from build123d import *

# Parameters (mm, degrees)
SKETCH3_R = 0.5


with BuildPart() as part:
    # Sweep2: sweep along a path in Sketch1
    with BuildLine(Plane(origin=(0, 0, 0), x_dir=(0, 0, -1), z_dir=(1, 0, 0))) as sweep2_path:
        Line((16, 4), (14, 4))
        ThreePointArc((14, 4), (13.292893219, 3.707106781), (13, 3))
        Line((13, 3), (13, 1))
        ThreePointArc((13, 1), (12.707106781, 0.292893219), (12, 0))
        Line((12, 0), (-12, 0))
        ThreePointArc((-12, 0), (-12.707106781, 0.292893219), (-13, 1))
        Line((-13, 1), (-13, 7))
        ThreePointArc((-13, 7), (-12.707106781, 7.707106781), (-12, 8))
        Line((-12, 8), (-6, 8))
    # Sketch3 → Sweep2 (sweep)
    with BuildSketch(Plane.XY):
        Circle(SKETCH3_R)
    sweep(path=sweep2_path.line)


solid = part.part
Work out the finished part from the listing and answer in its coordinate system (mm). A direction names the side the tool comes from. Give positions to 0.01 mm unless a question says otherwise; leave off trailing zeros. Order: outer loops, then holes, each group sorted by start corner. A loop starts at its lowest first (then second) coordinate and runs counter-clockwise, first axis right, second up. Notation, with made-up numbers: (68, -21) -> (95, -21) arc R26 ccw to (95, 6) -> close; hole circle Ø4 at (0, 46). An arc over 180 degrees is marked (long way). Answer as a JSON object with one key per item and string values. Group by question number.
1. Section B-B on y = 1.75 is taken. Determine the outline of the cut face in (x, z).
2. A tool of negligible diameter and unlimited length cuts with its end or side. For faces 4 (the cylindrical face through (-0.065, 4.496, -14.986)), 5 (the flat face through (0, 4, -16)), 6 (the cylindrical face through (0.231, 1.986, -13.444)), from which of +Z, -Z, +X, -X, +Y, -Y can it reach the whole face along a straight path? Write none if from no direction.
3. Section D-D on y = 5 is taken. Determine the outline of the cut face in (x, z), plus the area to 3 significant figures.
4. The mould has two halves that part along Z. Classify faces 1 (the cylindrical face through (-0.108, 8.488, 8.958)), 2 (the flat face through (0, 8, 6)), 3 (the cylindrical face through (-0.108, -0.488, 0.168)): released by +Z, released by -Z, zero draft, split by the parting line, or undercut.
5. Section A-A on x = 0 is taken. Determine the outline of the cut face in (y, z).
6. Consider line 1 along Y through (x, z) = (-0.05, 11.5); line 2 along Z through (x, y) = (0.05, 6.75); line 3 along Y through (x, z) = (0, -4). Determine where each line is inside the solid, lowest interval first. Write a range as [from, to].
7. A flat-ended cylindrical pin translates along its axis: pin 1 Ø1.5 at (y, z) = (4.5, -11.5) entering from +X. Find the tip coordinate at first contact, or state that the pin passes through.
8. Section C-C on z = -10.5 is taken. Determine the outline of the cut face in (x, y), plus the area to 3 significant figures.
Result sheet:
{
 "1": {"outline": "circle Ø1 at (0, -13); circle Ø1 at (0, 13)"},
 "2": {"face 4": "-Z", "face 5": "-Z, +X, -X, +Y, -Y", "face 6": "none"},
 "3": {"outline": "circle Ø1 at (0, 13)", "area": "0.785 mm^2"},
 "4": {"face 1": "zero draft", "face 2": "released by -Z", "face 3": "undercut"},
 "5": {"outline": "(-0.5, -12) arc R1.5 ccw to (1, -13.5) -> (3, -13.5) arc R0.5 cw to (3.5, -14) -> (3.5, -16) -> (4.5, -16) -> (4.5, -14) arc R1.5 ccw to (3, -12.5) -> (1, -12.5) arc R0.5 cw to (0.5, -12) -> (0.5, 12) arc R0.5 cw to (1, 12.5) -> (7, 12.5) arc R0.5 cw to (7.5, 12) -> (7.5, 6) -> (8.5, 6) -> (8.5, 12) arc R1.5 ccw to (7, 13.5) -> (1, 13.5) arc R1.5 ccw to (-0.5, 12) -> close"},
 "6": {"line 1": "y = [-0.5, 0.5], [7.5, 8.5]", "line 2": "z = [12.5, 13.5]", "line 3": "y = [-0.5, 0.5]"},
 "7": {"pin 1": "passes through"},
 "8": {"outline": "circle Ø1 at (0, 0)", "area": "0.785 mm^2"}
}
